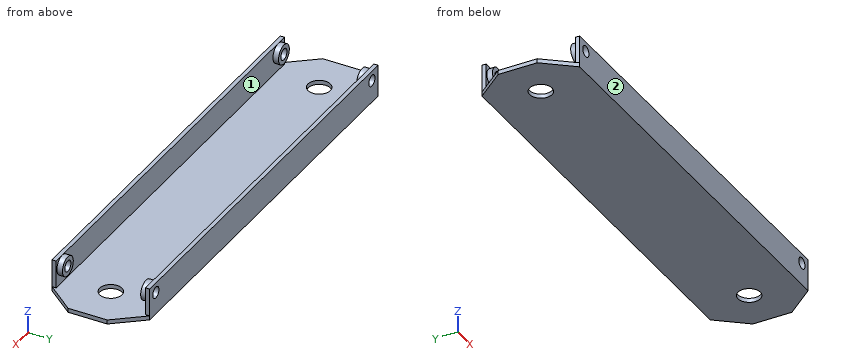
from build123d import *

# Parameters (mm, degrees)
SALIENTE_EXTRUIR1_DEPTH = 1.5
CROQUIS4_W              = 148
CROQUIS4_H              = 1.5
SALIENTE_EXTRUIR2_DEPTH = 10
CROQUIS5_W              = 148
CROQUIS5_H              = 1.5
SALIENTE_EXTRUIR3_DEPTH = 10
CROQUIS6_R              = 2
CORTAR_EXTRUIR6_DEPTH   = 3.5
CROQUIS9_R              = 3.5
SALIENTE_EXTRUIR5_DEPTH = 2
CROQUIS11_R             = 2
CORTAR_EXTRUIR7_DEPTH   = 2
CROQUIS12_R             = 3.5
SALIENTE_EXTRUIR6_DEPTH = 2
CROQUIS13_R             = 2
CORTAR_EXTRUIR8_DEPTH   = 2
CORTAR_EXTRUIR9_REACH   = 37
CROQUIS14_R             = 2
CROQUIS15_R             = 3.5
SALIENTE_EXTRUIR7_DEPTH = 2
CROQUIS16_R             = 2
CORTAR_EXTRUIR10_DEPTH  = 2
CORTAR_EXTRUIR11_REACH  = 37
CROQUIS17_R             = 2
CROQUIS18_R             = 3.5
SALIENTE_EXTRUIR8_DEPTH = 2
CROQUIS19_R             = 2
CORTAR_EXTRUIR12_DEPTH  = 2
CORTAR_EXTRUIR13_REACH  = 3.5
CROQUIS20_R             = 4


with BuildPart() as part:
    # Croquis1 → Saliente-Extruir1 (new body)
    with BuildSketch(Plane.XY):
        Polygon((110.114969998, 26.806936713), (118.614969998, 16.306936713), (118.614969998, 2.306936713), (110.114969998, -8.193063287), (-37.885030002, -8.193063287), (-46.385030002, 2.306936713), (-46.385030002, 16.306936713), (-37.885030002, 26.806936713), align=None)
    extrude(amount=SALIENTE_EXTRUIR1_DEPTH)

    # Croquis4 → Saliente-Extruir2 (add)
    with BuildSketch(Plane.XY.offset(1.5)):
        with Locations((36.114969998, 26.056936713)):
            Rectangle(CROQUIS4_W, CROQUIS4_H)
    extrude(amount=SALIENTE_EXTRUIR2_DEPTH)

    # Croquis5 → Saliente-Extruir3 (add)
    with BuildSketch(Plane.XY.offset(1.5)):
        with Locations((36.114969998, -7.443063287)):
            Rectangle(CROQUIS5_W, CROQUIS5_H)
    extrude(amount=SALIENTE_EXTRUIR3_DEPTH)

    # Croquis6 → Cortar-Extruir6 (cut)
    with BuildSketch(Plane(origin=(0, 26.806936713, 0), x_dir=(1, 0, 0), z_dir=(0, 1, 0))):
        with Locations((106.114969998, -8)):
            Circle(CROQUIS6_R)
        with Locations((-33.885030002, -8)):
            Circle(CROQUIS6_R)
    extrude(amount=-CORTAR_EXTRUIR6_DEPTH, mode=Mode.SUBTRACT)

    # Croquis9 → Saliente-Extruir5 (add)
    with BuildSketch(Plane.XZ.offset(-25.306936713)):
        with Locations((-33.885030002, 8)):
            Circle(CROQUIS9_R)
    extrude(amount=SALIENTE_EXTRUIR5_DEPTH)

    # Croquis11 → Cortar-Extruir7 (cut)
    with BuildSketch(Plane.XZ.offset(-23.306936713)):
        with Locations((-33.885030002, 8)):
            Circle(CROQUIS11_R)
    extrude(amount=-CORTAR_EXTRUIR7_DEPTH, mode=Mode.SUBTRACT)

    # Croquis12 → Saliente-Extruir6 (add)
    with BuildSketch(Plane.XZ.offset(-25.306936713)):
        with Locations((106.114969998, 8)):
            Circle(CROQUIS12_R)
    extrude(amount=SALIENTE_EXTRUIR6_DEPTH)

    # Croquis13 → Cortar-Extruir8 (cut)
    with BuildSketch(Plane.XZ.offset(-23.306936713)):
        with Locations((106.114969998, 8)):
            Circle(CROQUIS13_R)
    extrude(amount=-CORTAR_EXTRUIR8_DEPTH, mode=Mode.SUBTRACT)

    # Croquis14 → Cortar-Extruir9 (cut, up to next)
    with BuildSketch(Plane.XZ.offset(8.193063287), mode=Mode.PRIVATE) as cortar_extruir9_sk1:
        with Locations((-33.885030002, 8)):
            Circle(CROQUIS14_R)
    cortar_extruir9_tool1 = extrude(cortar_extruir9_sk1.sketch, amount=-CORTAR_EXTRUIR9_REACH, mode=Mode.PRIVATE) & part.part
    add(cortar_extruir9_tool1.solids().sort_by_distance((-33.88503, -8.193063, 8))[0], mode=Mode.SUBTRACT)

    # Croquis15 → Saliente-Extruir7 (add)
    with BuildSketch(Plane(origin=(0, -6.693063287, 0), x_dir=(1, 0, 0), z_dir=(0, 1, 0))):
        with Locations((-33.885030002, -8)):
            Circle(CROQUIS15_R)
    extrude(amount=SALIENTE_EXTRUIR7_DEPTH)

    # Croquis16 → Cortar-Extruir10 (cut)
    with BuildSketch(Plane(origin=(0, -4.693063287, 0), x_dir=(1, 0, 0), z_dir=(0, 1, 0))):
        with Locations((-33.885030002, -8)):
            Circle(CROQUIS16_R)
    extrude(amount=-CORTAR_EXTRUIR10_DEPTH, mode=Mode.SUBTRACT)

    # Croquis17 → Cortar-Extruir11 (cut, up to next)
    with BuildSketch(Plane.XZ.offset(8.193063287), mode=Mode.PRIVATE) as cortar_extruir11_sk1:
        with Locations((106.114969998, 8)):
            Circle(CROQUIS17_R)
    cortar_extruir11_tool1 = extrude(cortar_extruir11_sk1.sketch, amount=-CORTAR_EXTRUIR11_REACH, mode=Mode.PRIVATE) & part.part
    add(cortar_extruir11_tool1.solids().sort_by_distance((106.11497, -8.193063, 8))[0], mode=Mode.SUBTRACT)

    # Croquis18 → Saliente-Extruir8 (add)
    with BuildSketch(Plane(origin=(0, -6.693063287, 0), x_dir=(1, 0, 0), z_dir=(0, 1, 0))):
        with Locations((106.114969998, -8)):
            Circle(CROQUIS18_R)
    extrude(amount=SALIENTE_EXTRUIR8_DEPTH)

    # Croquis19 → Cortar-Extruir12 (cut)
    with BuildSketch(Plane(origin=(0, -4.693063287, 0), x_dir=(1, 0, 0), z_dir=(0, 1, 0))):
        with Locations((106.114969998, -8)):
            Circle(CROQUIS19_R)
    extrude(amount=-CORTAR_EXTRUIR12_DEPTH, mode=Mode.SUBTRACT)

    # Croquis20 → Cortar-Extruir13 (cut, up to next)
    with BuildSketch(Plane.XY.offset(1.5), mode=Mode.PRIVATE) as cortar_extruir13_sk1:
        with Locations((-31.385030002, 9.306936713)):
            Circle(CROQUIS20_R)
    cortar_extruir13_tool1 = extrude(cortar_extruir13_sk1.sketch, amount=-CORTAR_EXTRUIR13_REACH, mode=Mode.PRIVATE) & part.part
    add(cortar_extruir13_tool1.solids().sort_by_distance((-31.38503, 9.306937, 1.5))[0], mode=Mode.SUBTRACT)
    # Croquis20 → Cortar-Extruir13 (cut, up to next)
    with BuildSketch(Plane.XY.offset(1.5), mode=Mode.PRIVATE) as cortar_extruir13_sk2:
        with Locations((103.614969998, 9.306936713)):
            Circle(CROQUIS20_R)
    cortar_extruir13_tool2 = extrude(cortar_extruir13_sk2.sketch, amount=-CORTAR_EXTRUIR13_REACH, mode=Mode.PRIVATE) & part.part
    add(cortar_extruir13_tool2.solids().sort_by_distance((103.61497, 9.306937, 1.5))[0], mode=Mode.SUBTRACT)


solid = part.part
Design review of the part built by this model. Coordinates are the model's own, in mm. Face numbers are marked on the shaded views. Give positions to 0.01 mm unless a question says otherwise; leave off trailing zeros. Loops run counter-clockwise (first coordinate to the right, second up) from the corner with the lowest first, then second, coordinate; pieces in that order, holes last. Notation, with made-up numbers: M 47,-19.5 L 56,-19.5 A25 ccw 56,6.5 Z; hole C 29.5,-35.75 d9. An arc over 180 degrees is marked long. Write item = value, one per line.
Q1. We need section D-D (y = -2.5). Give the boundary of the cut face in (x, z), plus the area to 3 significant figures.
Output values:
outline = M -42.49,0 L 114.72,0 L 114.72,1.5 L -42.49,1.5 Z
area = 236 mm^2
Q2. Draft analysis for pull direction X (two halves, no side actions). For the marked faces 1 and 2, state which applies: +X half, -X half, draft (parallel to the pull), parting line (faces both ways), or undercut.
Output values:
face_1 = undercut
face_2 = draft
Q3. We need section C-C (y = 20.5). Give the boundary of the cut face in (x, z).
Output values:
outline = M -42.99,0 L 115.22,0 L 115.22,1.5 L -42.99,1.5 Z
Q4. We need section B-B (z = 8). Count the separate pieces of the cut face and the enclosed holes in it, plus the area to 3 significant figures.
Output values:
separate_pieces = 6
enclosed_holes = 0
area = 444 mm^2
Q5. To check wall thickness, follow line 1 (X direction, y = -7.3, z = 8); line 2 (X direction, y = 24, z = 8); line 3 (Y direction, x = 108, z = 9). State the ranges of each line that lie inside material, in increasing order. Write a range as [from, to].
Output values:
line_1 = [-37.89, -35.89], [-31.89, 104.11], [108.11, 110.11]
line_2 = [-37.39, -35.89], [-31.89, -30.39], [102.61, 104.11], [108.11, 109.61]
line_3 = [-8.19, -4.69], [23.31, 26.81]
Q6. We need section A-A (x = 83). Give the boundary of the cut face in (y, z), plus the area to 3 significant figures.
Output values:
outline = M -8.19,0 L 26.81,0 L 26.81,11.5 L 25.31,11.5 L 25.31,1.5 L -6.69,1.5 L -6.69,11.5 L -8.19,11.5 Z
area = 82.5 mm^2
Q7. Insertion check: pin 1 (10.5 mm diameter, centred on x = 3, y = 10.5, fed in from +Z); pin 2 (0.8 mm diameter, centred on y = 26, z = 7, fed in from +X) (3 decimals); pin 3 (0.5 mm diameter, centred on y = -7.5, z = 6.5, fed in from -X). Each pin has a flat end and moves straight along its axis. Give the tip position at first contact, or say it passes through.
Output values:
pin_1 = 1.5
pin_2 = 110.115
pin_3 = -37.89
